from build123d import *

# Parameters (mm, degrees)
BOSS_EXTRUDE1_DEPTH = 2
CUT_EXTRUDE1_DEPTH  = 2
SKETCH3_R           = 12
BOSS_EXTRUDE2_DEPTH = 2
SKETCH4_W           = 30
SKETCH4_H           = 30
BOSS_EXTRUDE3_DEPTH = 2
SKETCH5_R           = 2
BOSS_EXTRUDE4_DEPTH = 4.5
SKETCH6_R           = 2
BOSS_EXTRUDE5_DEPTH = 30
SKETCH7_R           = 20
BOSS_EXTRUDE6_DEPTH = 10
FILLET1_R           = 5


with BuildPart() as part:
    # Sketch1 → Boss-Extrude1 (new body)
    with BuildSketch(Plane(origin=(0, 0, 0), x_dir=(1, 0, 0), z_dir=(0, 1, 0))):
        with BuildLine():
            Line((25, -20), (-25, -20))
            ThreePointArc((-25, -20), (-28.535533906, -18.535533906), (-30, -15))
            Line((-30, -15), (-30, 15))
            ThreePointArc((-30, 15), (-28.535533906, 18.535533906), (-25, 20))
            Line((-25, 20), (25, 20))
            ThreePointArc((25, 20), (28.535533906, 18.535533906), (30, 15))
            Line((30, 15), (30, -15))
            ThreePointArc((30, -15), (28.535533906, -18.535533906), (25, -20))
        make_face()
    extrude(amount=BOSS_EXTRUDE1_DEPTH)

    # Sketch2 → Cut-Extrude1 (cut)
    with BuildSketch(Plane(origin=(0, 2, 0), x_dir=(1, 0, 0), z_dir=(0, 1, 0))):
        with BuildLine():
            Line((-25, 17), (-20, 17))
            ThreePointArc((-20, 17), (-18, 15), (-20, 13))
            Line((-20, 13), (-25, 13))
            ThreePointArc((-25, 13), (-27, 15), (-25, 17))
        make_face()
        with BuildLine():
            Line((25, 17), (20, 17))
            ThreePointArc((20, 17), (18, 15), (20, 13))
            Line((20, 13), (25, 13))
            ThreePointArc((25, 13), (27, 15), (25, 17))
        make_face()
        with BuildLine():
            Line((25, -17), (20, -17))
            ThreePointArc((20, -17), (18, -15), (20, -13))
            Line((20, -13), (25, -13))
            ThreePointArc((25, -13), (27, -15), (25, -17))
        make_face()
        with BuildLine():
            Line((-25, -17), (-20, -17))
            ThreePointArc((-20, -17), (-18, -15), (-20, -13))
            Line((-20, -13), (-25, -13))
            ThreePointArc((-25, -13), (-27, -15), (-25, -17))
        make_face()
    extrude(amount=-CUT_EXTRUDE1_DEPTH, mode=Mode.SUBTRACT)

    # Sketch3 → Boss-Extrude2 (add)
    with BuildSketch(Plane.XZ):
        with Locations(Location((0, 0, 0), (0, 0, 270))):
            Circle(SKETCH3_R)
    extrude(amount=BOSS_EXTRUDE2_DEPTH)

    # Sketch4 → Boss-Extrude3 (add)
    with BuildSketch(Plane.XZ.offset(2)):
        Rectangle(SKETCH4_W, SKETCH4_H)
    extrude(amount=BOSS_EXTRUDE3_DEPTH)

    # Sketch5 → Boss-Extrude4 (add)
    with BuildSketch(Plane.XY.offset(15)):
        with BuildLine():
            Line((-15, -4), (6.939310229, -42))
            ThreePointArc((6.939310229, -42), (7.671361037, -42.732050808), (8.671361037, -43))
            Line((8.671361037, -43), (13, -43))
            ThreePointArc((13, -43), (14.414213562, -42.414213562), (15, -41))
            Line((15, -41), (15, -4))
            Line((15, -4), (-15, -4))
        make_face()
        with Locations((10.835680518, -38)):
            Circle(SKETCH5_R, mode=Mode.SUBTRACT)
    boss_extrude4 = extrude(amount=-BOSS_EXTRUDE4_DEPTH)

    # Mirror1: Boss-Extrude4 across plane
    add(boss_extrude4.mirror(Plane.XY))

    # Sketch6 → Boss-Extrude5 (add)
    with BuildSketch(Plane.XY.offset(15)):
        with Locations((10.835680518, -38)):
            Circle(SKETCH6_R)
    extrude(amount=-BOSS_EXTRUDE5_DEPTH)

    # Sketch7 → Boss-Extrude6 (add, symmetric)
    with BuildSketch(Plane.XY):
        with Locations((10.835680518, -38)):
            Circle(SKETCH7_R)
    extrude(amount=BOSS_EXTRUDE6_DEPTH, both=True)

    # Fillet1
    fillet1_edges = [part.edges().sort_by_distance(p)[0] for p in [
        (-9.164319482, -38, -10),
        (-9.164319482, -38, 10),
    ]]
    fillet(fillet1_edges, radius=FILLET1_R)


solid = part.part
Check sheet for the modelled part. Datum: model origin and axes. Units: mm. A direction names the side the tool comes from. Round coordinates to 2 decimals unless told otherwise and drop trailing zeros. Loops run counter-clockwise (first coordinate to the right, second up) from the corner with the lowest first, then second, coordinate; pieces in that order, holes last. Notation, with made-up numbers: (18.25, 41) -> (73.25, 41) arc R13 ccw to (73.25, 57) -> close; hole circle Ø2 at (89.5, 60.25). An arc over 180 degrees is marked (long way). Put each result on its own line as item: value. Start each with the question number.
1. Section check B-B (y = -14). Enter the section's corners in (x, z), plus the area to 3 significant figures.
2. Section check D-D (x = 23). Give the number of separate pieces and of enclosed holes in the cut face, plus the area to 3 significant figures.
3. Scan lines: probe 1 along Z at (x, y) = (-7.5, -14); probe 2 along Y at (x, z) = (14, 2); probe 3 along Z at (x, y) = (0.5, -3.5). Record each from-to range of solid material in increasing order.
4. Section check A-A (z = 0). Enter the section's corners in (x, y).
5. Gauge pin test, flat ends, axial feed: pin 1 (24 mm diameter, centred on x = 16.5, y = -37.5, fed in from +Z); pin 2 (2 mm diameter, centred on x = 10.5, z = -12, fed in from -Y); pin 3 (1 mm diameter, centred on y = 0.5, z = 4, fed in from +X). Record the tip position at first contact, or that the pin passes through.
6. Draft check along X on faces 1 (the face through (0, 1, -20)), 2 (the face through (10.4, -39.95, -10.25)), 3 (the face through (-18, 1, 15)). Enter one of: +X half, -X half, draft (parallel to the pull), parting line (faces both ways), or undercut.
7. Access from +Z, -Z, +X, -X, +Y, -Y to the whole of each face (thin tool, end or side, straight path). Record for faces 4 (the face through (14.4, -42.43, -12.78)), 5 (the face through (18, 1, 15)), 6 (the face through (3, -18, 15)), 7 (the face through (11, -43, -13)).
8. Section check C-C (z = 16). Enter the section's corners in (x, y), plus the area to 3 significant figures.
Findings:
1. outline: (-9.23, -15) -> (15, -15) -> (15, -10.5) -> (-9.23, -10.5) -> close; (-9.23, 10.5) -> (15, 10.5) -> (15, 15) -> (-9.23, 15) -> close
1. area: 218 mm^2
2. separate pieces: 4
2. enclosed holes: 0
2. area: 671 mm^2
3. probe 1: z = -15 to -10.5, 10.5 to 15
3. probe 2: y = -57.75 to -18.25, -4 to -2, 0 to 2
3. probe 3: z = -15 to 15
4. outline: (-30, 0) -> (-12, 0) -> (-12, -2) -> (-15, -2) -> (-15, -4) -> (15, -4) -> (15, -2) -> (12, -2) -> (12, 0) -> (30, 0) -> (30, 2) -> (-30, 2) -> close; circle Ø40 at (10.84, -38)
5. pin 1: stops at z = 15
5. pin 2: stops at y = -43
5. pin 3: stops at x = 30
6. face 1: draft
6. face 2: parting line
6. face 3: undercut
7. face 4: -Z, +X, -Y
7. face 5: +Y, -Y
7. face 6: +Z, +X, -X, -Y
7. face 7: -Z, +X, -X, -Y
8. outline: (-29.9, 0) -> (-26.73, 0) -> (-26.73, 2) -> (-29.9, 2) -> close; (-18.27, 0) -> (18.27, 0) -> (18.27, 2) -> (-18.27, 2) -> close; (26.73, 0) -> (29.9, 0) -> (29.9, 2) -> (26.73, 2) -> close
8. area: 85.7 mm^2
